Here's the drawing with two shaded views (mm, measured from the low corner). I have some questions. A direction names the side the tool comes from. Round coordinates to 2 decimals unless told otherwise and drop trailing zeros. Write each loop counter-clockwise with the first axis right and the second up, starting at its lowest first coordinate (ties: lowest second). Pieces come first, ordered by that corner, then holes. Notation, with made-up numbers: M 67,35 L 80,35 A22 cw 80,42 Z; hole C 47,25.5 d8. An arc over 180 degrees is marked long. Answer as a JSON object with one key per item and string values. Group by question number.
1) If we mould it in two halves opening along Y, with no side actions, what happens to the marked faces 3, 4, 5 and 6? For each: +Y half, -Y half, draft (parallel to the pull), parting line (faces both ways), or undercut.
2) Please list where these lines run through material, in increasing order: L1, parallel to X at y = 57, z = 38; L2, parallel to Y at x = 17, z = 59; L3, parallel to X at y = 52, z = 11.5. Write a range as [from, to].
3) Suppose I cut it at D-D, the plane x = 63.5. Write out the boundary of the cut face in (y, z).
4) On a 3-axis mill with a long thin cutter (end or side, diameter ignored), from which of +Z, -Z, +X, -X, +Y, -Y can I reach the whole of each face in a straight line? I mean the marked faces 1 and 2. Say none if no direction works.
5) Suppose I cut it at B-B, the plane x = 109.22. Write out the boundary of the cut face in (y, z).
6) Suppose I cut it at A-A, the plane y = 57.15. Write out the boundary of the cut face in (x, z).
7) I'm going to push flat-ended pins straight in: pin 1 Ø8 at (x, z) = (53, 49.5) entering from +Y; pin 2 Ø1.5 at (x, z) = (73, 74.5) entering from -Y; pin 3 Ø4 at (x, y) = (52, 14) entering from +Z; pin 4 Ø8 at (x, z) = (29, 22) entering from -Y. Where does each tip first touch, or does it pass through?
8) Suppose I cut it at C-C, the plane z = 61. Write out the boundary of the cut face in (x, y), and give its area (3 significant figures).
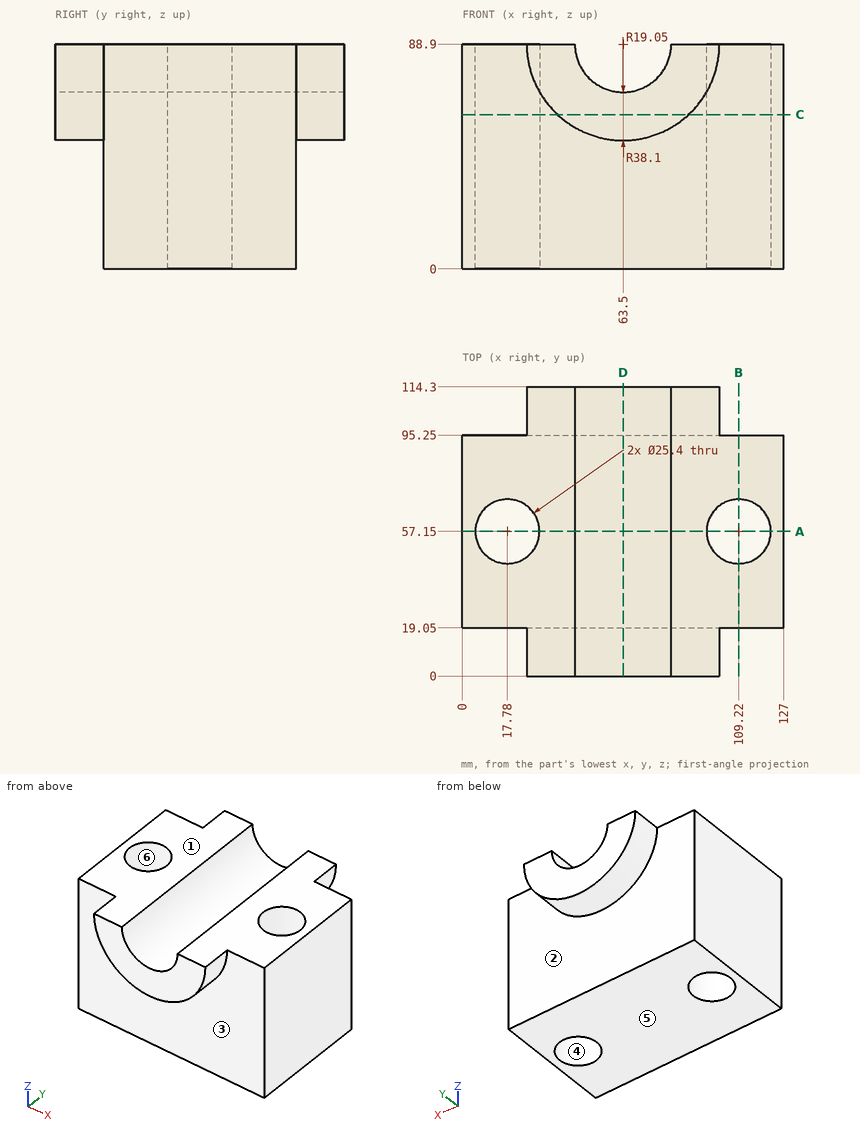
Results:
{
 "1": {"face 3": "-Y half", "face 4": "undercut", "face 5": "draft", "face 6": "undercut"},
 "2": {"L1": "[0, 5.08], [30.48, 96.52], [121.92, 127]", "L2": "[19.05, 44.47], [69.83, 95.25]", "L3": "[0, 6.17], [29.39, 97.61], [120.83, 127]"},
 "3": {"outline": "M 0,50.8 L 19.05,50.8 L 19.05,0 L 95.25,0 L 95.25,50.8 L 114.3,50.8 L 114.3,69.85 L 0,69.85 Z"},
 "4": {"face 1": "+Z, +X, -X, +Y, -Y", "face 2": "-Z, +Y"},
 "5": {"outline": "M 19.05,0 L 44.45,0 L 44.45,88.9 L 19.05,88.9 Z; M 69.85,0 L 95.25,0 L 95.25,88.9 L 69.85,88.9 Z"},
 "6": {"outline": "M 0,0 L 5.08,0 L 5.08,88.9 L 0,88.9 Z; M 30.48,0 L 96.52,0 L 96.52,88.9 L 82.55,88.9 A19.05 cw 44.45,88.9 L 30.48,88.9 Z; M 121.92,0 L 127,0 L 127,88.9 L 121.92,88.9 Z"},
 "7": {"pin 1": "y = 114.3", "pin 2": "through", "pin 3": "z = 75.46", "pin 4": "y = 19.05"},
 "8": {"outline": "M 0,19.05 L 37.55,19.05 L 37.55,0 L 89.45,0 L 89.45,19.05 L 127,19.05 L 127,95.25 L 89.45,95.25 L 89.45,114.3 L 37.55,114.3 L 37.55,95.25 L 0,95.25 Z; hole C 17.78,57.15 d25.4; hole C 109.22,57.15 d25.4", "area": "10,600 mm^2"}
}
